CAD build for the part. Positions are in the model's coordinates, mm. Face numbers are marked on the shaded views. Give positions to 0.01 mm unless a question says otherwise; leave off trailing zeros. Loops run counter-clockwise (first coordinate to the right, second up) from the corner with the lowest first, then second, coordinate; pieces in that order, holes last.
```python
from build123d import *

# Parameters (mm, degrees)
F0_R      = 2
F1_DEPTH  = 10
F3_R      = 1
F4_DEPTH  = 5
F5_R      = 0.5
F6_DEPTH  = 104.53913
F7_R      = 0.5
F8_DEPTH  = 94.789131
F9_R      = 0.5
F10_DEPTH = 68.501


with BuildPart() as f1:
    # F0 (on Top) → F1 (new body)
    with BuildSketch(Plane.XY):
        with BuildLine():
            Line((36.661742, -24.5), (41.431151, -16.239141))
            ThreePointArc((41.431151, -16.239141), (44.5, 0), (41.431151, 16.239141))
            Line((41.431151, 16.239141), (34.779084, 27.760859))
            ThreePointArc((34.779084, 27.760859), (22.25, 38.53813), (6.652067, 44))
            Line((6.652067, 44), (-6.652067, 44))
            ThreePointArc((-6.652067, 44), (-22.25, 38.53813), (-34.779084, 27.760859))
            Line((-34.779084, 27.760859), (-41.431151, 16.239141))
            ThreePointArc((-41.431151, 16.239141), (-44.5, 0), (-41.431151, -16.239141))
            Line((-41.431151, -16.239141), (-36.661742, -24.5))
            Line((-36.661742, -24.5), (36.661742, -24.5))
        make_face()
        with Locations((-34.641016, -20)):
            Circle(F0_R, mode=Mode.SUBTRACT)
        with Locations((0, -20)):
            Circle(F0_R, mode=Mode.SUBTRACT)
        with Locations((34.641016, -20)):
            Circle(F0_R, mode=Mode.SUBTRACT)
        with Locations((-34.641016, 20)):
            Circle(F0_R, mode=Mode.SUBTRACT)
        with BuildLine():
            Line((31.937439, -15.5), (-31.937439, -15.5))
            ThreePointArc((-31.937439, -15.5), (0, 35.5), (31.937439, -15.5))
        make_face(mode=Mode.SUBTRACT)
        with Locations((0, 40)):
            Circle(F0_R, mode=Mode.SUBTRACT)
        with Locations((34.641016, 20)):
            Circle(F0_R, mode=Mode.SUBTRACT)
    extrude(amount=F1_DEPTH)

    # F3 (on face) → F4 (cut)
    with BuildSketch(Plane(origin=(0, -17.25, 17.25), x_dir=(1, 0, 0), z_dir=(0, -0.707107, 0.707107))):
        with Locations((-34.641016, -10.253048)):
            Circle(F3_R)
        with Locations((34.641016, -10.253048)):
            Circle(F3_R)
    extrude(amount=-F4_DEPTH, mode=Mode.SUBTRACT)

    # F5 (on face) → F6 (cut, through all)
    with BuildSketch(Plane(origin=(38.105118, -22, 0), x_dir=(0.5, 0.866025, 0), z_dir=(0.866025, -0.5, 0))):
        with Locations((0, 5)):
            Circle(F5_R)
    extrude(amount=-F6_DEPTH, mode=Mode.SUBTRACT)

    # F7 (on face) → F8 (cut, through all)
    with BuildSketch(Plane(origin=(38.105118, 22, 0), x_dir=(-0.5, 0.866025, 0), z_dir=(0.866025, 0.5, 0))):
        with Locations((0, 5)):
            Circle(F7_R)
    extrude(amount=-F8_DEPTH, mode=Mode.SUBTRACT)

    # F9 (on face) → F10 (cut, through all)
    with BuildSketch(Plane(origin=(0, 44, 0), x_dir=(-1, 0, 0), z_dir=(0, 1, 0))):
        with Locations((0, 5)):
            Circle(F9_R)
    extrude(amount=-F10_DEPTH, mode=Mode.SUBTRACT)


solid = f1.part
```
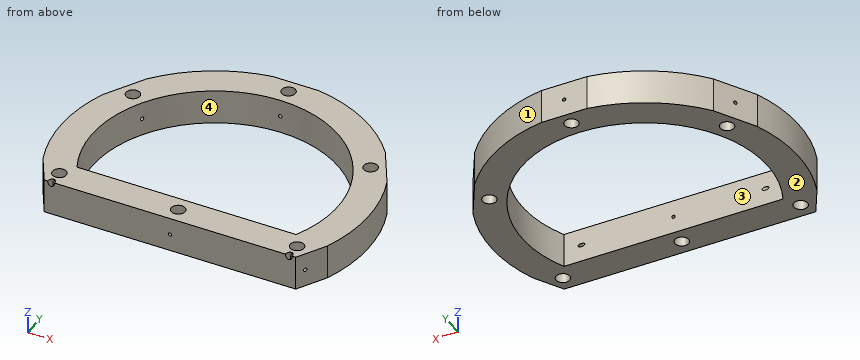
1. Saw through at C-C, the plane x = 20. List the corners of the cut face in (y, z), and give its area (3 significant figures).
Responses:
outline: (-24.5, 0) - (-15.5, 0) - (-15.5, 10) - (-24.5, 10) - close; (29.33, 0) - (39.75, 0) - (39.75, 10) - (29.33, 10) - close
area: 194 mm2
2. Saw through at A-A, the plane y = 40. List the corners of the cut face in (x, z), and give its area (3 significant figures).
Responses:
outline: (-19.5, 0) - (-2, 0) - (-2, 10) - (-19.5, 10) - close; (2, 0) - (19.5, 0) - (19.5, 10) - (2, 10) - close
area: 350 mm2
3. Pull direction Y, two halves, no side cores. Call the marked faces 1, 2, 3 and 4: released by +Y, released by -Y, zero draft, split by the parting line, or undercut.
Responses:
face 1: released by +Y
face 2: zero draft
face 3: undercut
face 4: undercut
4. Probe line 1 along Y through (x, z) = (0, 5.75); line 2 along Y through (x, z) = (25, 8.75); line 3 along Y through (x, z) = (36, 4.5). List the from-to ranges inside material, lowest first.
Responses:
line 1: y = -24.5 to -22, -18 to -15.5, 35.5 to 38, 42 to 44
line 2: y = -24.5 to -15.5, 25.2 to 36.81
line 3: y = -24.5 to -21.47, -18.53 to 18.53, 21.47 to 25.65
5. Drop flat-ended pins along their axis: pin 1 (4 mm diameter, centred on x = -16, z = 8.5, fed in from +Y); pin 2 (4.5 mm diameter, centred on x = 34.64, y = 20, fed in from -Z); pin 3 (6 mm diameter, centred on y = -13, z = 3.5, fed in from +X); pin 4 (1.5 mm diameter, centred on y = -5.5, z = 6.5, fed in from -X). Give the stop position or say it passes through.
Responses:
pin 1: stops at y = 42.24
pin 2: stops at z = 0
pin 3: stops at x = 43.36
pin 4: stops at x = -44.25
6. Saw through at B-B, the plane z = 3.5. List the corners of the cut face in (x, y).
Responses:
outline: (-41.43, -16.24) - (-36.66, -24.5) - (36.66, -24.5) - (41.43, -16.24) arc R44.5 ccw to (41.43, 16.24) - (34.78, 27.76) arc R44.5 ccw to (6.65, 44) - (-6.65, 44) arc R44.5 ccw to (-34.78, 27.76) - (-41.43, 16.24) arc R44.5 ccw to start; hole circle Ø4 at (-34.64, -20); hole circle Ø4 at (-34.64, 20); hole (-31.94, -15.5) - (31.94, -15.5) arc R35.5 ccw (long way) to start; hole circle Ø4 at (0, -20); hole circle Ø4 at (0, 40); hole circle Ø4 at (34.64, -20); hole circle Ø4 at (34.64, 20)
